Drawing for the job (mm, zero at the part's lowest x, y, z). A direction names the side the tool comes from. Give positions to 0.01 mm unless a question says otherwise; leave off trailing zeros. Write each loop counter-clockwise with the first axis right and the second up, starting at its lowest first coordinate (ties: lowest second). Pieces come first, ordered by that corner, then holes. Notation, with made-up numbers: M -5.5,66.25 L 20.5,66.25 A32 cw 20.5,99.25 Z; hole C 23,11 d7. An arc over 180 degrees is marked long. Use CSV: the item, a comma, the result in double quotes. Start each with the question number.
1. Drop flat-ended pins along their axis: pin 1 Ø22 at (y, z) = (82, 18.5) entering from -X; pin 2 Ø4 at (y, z) = (101, 28.5) entering from +X; pin 3 Ø22 at (x, y) = (22, 80) entering from -Z. Give the stop position or say it passes through.
2. Band-saw the part on C-C, the plane y = 10. List the corners of the cut face in (x, z), then the cut area to 3 significant figures.
3. Band-saw the part on A-A, the plane x = 28.5. List the corners of the cut face in (y, z), then the cut area to 3 significant figures.
4. Band-saw the part on D-D, the plane x = 8.5. List the corners of the cut face in (y, z).
5. 3-axis set-ups, long thin cutter, end or side, ignore diameter. For the marked faces 1, 2, 3 and 4: which of +Z, -Z, +X, -X, +Y, -Y reach the whole face in a straight line?
6. Drill centre lines: line 1 along Z through (x, y) = (27.5, 100.5); line 2 along Y through (x, z) = (11.5, 2.5). Where is each one in solid material? Low to high. Write a range as from..to.
7. Band-saw the part on B-B, the plane z = 22. List the corners of the cut face in (x, y), then the cut area to 3 significant figures.
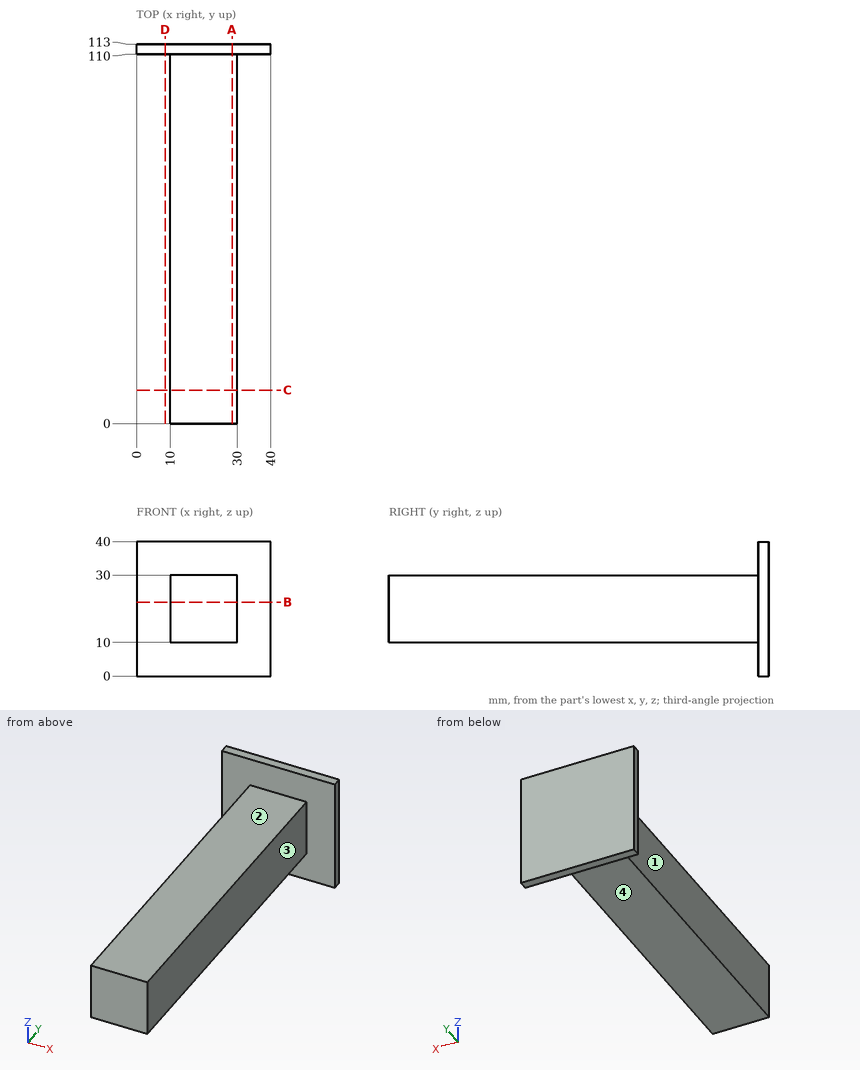
Output:
1,pin 1,"stops at x = 10"
1,pin 2,"stops at x = 30"
1,pin 3,"stops at z = 10"
2,outline,"M 10,10 L 30,10 L 30,30 L 10,30 Z"
2,area,"400 mm²"
3,outline,"M 0,10 L 110,10 L 110,0 L 113,0 L 113,40 L 110,40 L 110,30 L 0,30 Z"
3,area,"2,320 mm²"
4,outline,"M 110,0 L 113,0 L 113,40 L 110,40 Z"
5,face 1,"+Z, -Z, -X, -Y"
5,face 2,"+Z, +X, -X, -Y"
5,face 3,"+Z, -Z, +X, -Y"
5,face 4,"-Z, +X, -X, -Y"
6,line 1,"z = 10..30"
6,line 2,"y = 110..113"
7,outline,"M 0,110 L 10,110 L 10,0 L 30,0 L 30,110 L 40,110 L 40,113 L 0,113 Z"
7,area,"2,320 mm²"
